from build123d import *

# Parameters (mm, degrees)
SKETCH1_R               = 2.5
BOSS_EXTRUDE1_DEPTH     = 100
CUT_EXTRUDE1_DEPTH      = 5
BOSS_EXTRUDE2_DEPTH     = 1
CHAMFER1_SIZE           = 1
CUT_EXTRUDE2_DEPTH      = 3.5000001
CUT_EXTRUDE2_DEPTH_BACK = 3.5000001


with BuildPart() as part:
    # Sketch1 → Boss-Extrude1 (new body)
    with BuildSketch(Plane.XY):
        Circle(SKETCH1_R)
    extrude(amount=BOSS_EXTRUDE1_DEPTH)

    # Sketch2 → Cut-Extrude1 (cut, symmetric)
    with BuildSketch(Plane(origin=(0, 0, 0), x_dir=(0, 0, -1), z_dir=(1, 0, 0))):
        with BuildLine():
            Line((-94, 4), (-88, 4))
            ThreePointArc((-88, 4), (-87.292893219, 3.707106781), (-87, 3))
            Line((-87, 3), (-87, 2))
            ThreePointArc((-87, 2), (-87.292893219, 1.292893219), (-88, 1))
            Line((-88, 1), (-94, 1))
            ThreePointArc((-94, 1), (-94.707106781, 1.292893219), (-95, 2))
            Line((-95, 2), (-95, 3))
            ThreePointArc((-95, 3), (-94.707106781, 3.707106781), (-94, 4))
        make_face()
        with BuildLine():
            Line((-87, -3), (-87, -2))
            ThreePointArc((-87, -2), (-87.292893219, -1.292893219), (-88, -1))
            Line((-88, -1), (-94, -1))
            ThreePointArc((-94, -1), (-94.707106781, -1.292893219), (-95, -2))
            Line((-95, -2), (-95, -3))
            ThreePointArc((-95, -3), (-94.707106781, -3.707106781), (-94, -4))
            Line((-94, -4), (-88, -4))
            ThreePointArc((-88, -4), (-87.292893219, -3.707106781), (-87, -3))
        make_face()
    extrude(amount=CUT_EXTRUDE1_DEPTH, both=True, mode=Mode.SUBTRACT)

    # Sketch2_2 → Boss-Extrude2 (add, symmetric)
    with BuildSketch(Plane(origin=(0, 0, 0), x_dir=(0, 0, -1), z_dir=(1, 0, 0))):
        with BuildLine():
            Line((-94, 4), (-88, 4))
            ThreePointArc((-88, 4), (-87.292893219, 3.707106781), (-87, 3))
            Line((-87, 3), (-87, 2))
            ThreePointArc((-87, 2), (-87.292893219, 1.292893219), (-88, 1))
            Line((-88, 1), (-94, 1))
            ThreePointArc((-94, 1), (-94.707106781, 1.292893219), (-95, 2))
            Line((-95, 2), (-95, 3))
            ThreePointArc((-95, 3), (-94.707106781, 3.707106781), (-94, 4))
        make_face()
        with BuildLine():
            Line((-87, -3), (-87, -2))
            ThreePointArc((-87, -2), (-87.292893219, -1.292893219), (-88, -1))
            Line((-88, -1), (-94, -1))
            ThreePointArc((-94, -1), (-94.707106781, -1.292893219), (-95, -2))
            Line((-95, -2), (-95, -3))
            ThreePointArc((-95, -3), (-94.707106781, -3.707106781), (-94, -4))
            Line((-94, -4), (-88, -4))
            ThreePointArc((-88, -4), (-87.292893219, -3.707106781), (-87, -3))
        make_face()
    extrude(amount=BOSS_EXTRUDE2_DEPTH, both=True)

    # Chamfer1
    chamfer1_edges = [part.edges().sort_by_distance(p)[0] for p in [
        (-2.5, 0, 100),
    ]]
    chamfer(chamfer1_edges, length=CHAMFER1_SIZE)

    # Sketch3 → Cut-Extrude2 (cut, two sides)
    with BuildSketch(Plane(origin=(0, 0, 0), x_dir=(0, 0, -1), z_dir=(1, 0, 0))) as cut_extrude2_sk:
        Polygon((-15, 2.5), (0, 0.5), (0, 2.5), align=None)
        Polygon((0, -2.5), (0, -0.5), (-15, -2.5), align=None)
    extrude(amount=CUT_EXTRUDE2_DEPTH, mode=Mode.SUBTRACT)
    extrude(cut_extrude2_sk.sketch, amount=-CUT_EXTRUDE2_DEPTH_BACK, mode=Mode.SUBTRACT)


solid = part.part
Work out the finished part from the listing and answer in its coordinate system (mm). A direction names the side the tool comes from. Coordinates: 2 decimals unless noted, no trailing zeros. Order: outer loops, then holes, each group sorted by start corner. A loop starts at its lowest first (then second) coordinate and runs counter-clockwise, first axis right, second up. Notation, with made-up numbers: (8, -5.5) - (16, -5.5) arc R10 cw to (16, 11.5) - close; hole circle Ø8 at (-19.75, -38). An arc over 180 degrees is marked (long way). Put each result on its own line as item: value. Start each with the question number.
1) Flat-ended cylindrical pins translate along their axes: pin 1 (1.4 mm diameter, centred on x = 1.5, z = 90.5, fed in from -Y); pin 2 (3 mm diameter, centred on y = 2.5, z = 25, fed in from +X); pin 3 (3.5 mm diameter, centred on y = -2.5, z = 89, fed in from +X); pin 4 (2.5 mm diameter, centred on y = 3, z = 92.5, fed in from +X). Find the tip coordinate at first contact, or state that the pin passes through.
2) Find section B-B (z = 80.5). Give the vertices of the cut face in (x, y), plus the area to 3 significant figures.
3) Find section A-A (x = 0). Give the vertices of the cut face in (y, z).
4) For faces 5 (the flat face through (0.034, -1.264, 5.728)), 6 (the flat face through (-1, -2, 91)), 7 (the flat face through (0, -4, 91)), 8 (the flat face through (1, -2, 91)), 9 (the flat face through (1, 3, 91)), determine the directions among +Z, -Z, +X, -X, +Y, -Y from which every point of the face is accessible in a straight line to the end or side of a thin tool.
5) For a pull along Z with two mould halves and no side action, classify faces 1 (the flat face through (0, 0, 100)), 2 (the flat face through (-1, 3, 91)), 3 (the flat face through (-0.03, 1.29, 5.94)), 4 (the flat face through (0, 4, 91)) as released by +Z, released by -Z, zero draft, split by the parting line, or undercut.
6) Find the intervals of material crossed by line 1 (Z direction, x = -0.2, y = -3); line 2 (Y direction, x = 0.2, z = 67.5), in increasing order. Write a range as from..to.
Results list:
1. pin 1: stops at y = -4
1. pin 2: stops at x = 2.29
1. pin 3: stops at x = 2.38
1. pin 4: stops at x = 1
2. outline: circle Ø5 at (0, 0)
2. area: 19.6 mm^2
3. outline: (-4, 88) arc R1 ccw to (-3, 87) - (-2.5, 87) - (-2.5, 15) - (-0.5, 0) - (0.5, 0) - (2.5, 15) - (2.5, 87) - (3, 87) arc R1 ccw to (4, 88) - (4, 94) arc R1 ccw to (3, 95) - (2.5, 95) - (2.5, 99) - (1.5, 100) - (-1.5, 100) - (-2.5, 99) - (-2.5, 95) - (-3, 95) arc R1 ccw to (-4, 94) - close
4. face 5: -Z, +X, -X, -Y
4. face 6: -X, -Y
4. face 7: +Z, -Z, +X, -X, -Y
4. face 8: +X, -Y
4. face 9: +X, +Y
5. face 1: released by +Z
5. face 2: undercut
5. face 3: released by -Z
5. face 4: zero draft
6. line 1: z = 87..95
6. line 2: y = -2.49..2.49
